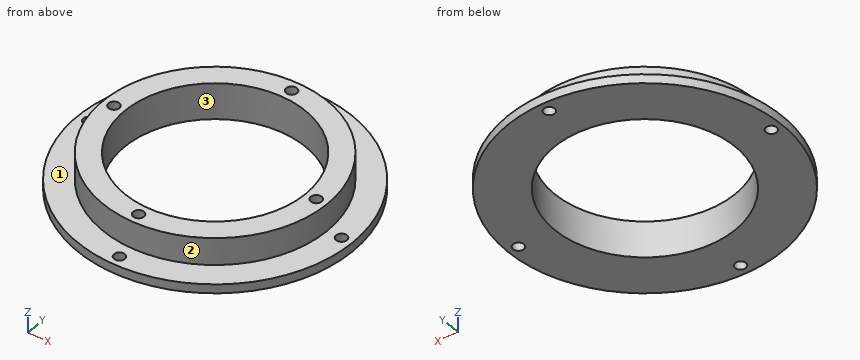
Autodesk Inventor part; units mm, degrees
ref_plane "YZ Plane" through (0, 0, 0) normal (1, 0, 0) x (0, 1, 0)
ref_plane "XZ Plane" through (0, 0, 0) normal (0, 1, 0) x (-1, 0, 0)
ref_plane "XY Plane" through (0, 0, 0) normal (0, 0, 1) x (1, 0, 0)
sketch "스케치1" plane through (0, 0, 0) normal (0, 0, 1) x (1, 0, 0)
  circle A0 centre (0, 0) radius 25
  circle A1 centre (-35, 0) radius 1.5
  circle A2 centre (0, 0) radius 31
  circle A3 centre (0, 0) radius 38
  circle A4 centre (0, -35) radius 1.5
  circle A5 centre (35, 0) radius 1.5
  circle A6 centre (0, 35) radius 1.5
  dimension "d0" = 50
  dimension "d2" = 3
  dimension "d4" = 6
  dimension "d27" = 1.5
  dimension "d28" = 35
  dimension "d31" = 360
extrude "돌출1" add sketch "스케치1" along normal blind 2.5 contours A3
extrude "돌출2" add sketch "스케치1" along normal blind 10 contours A2
sketch "스케치2" plane through (0, 0, 10) normal (0, 0, 1) x (1, 0, 0)
  circle A0 centre (0, 0) radius 25
  circle A1 centre (0, 0) radius 31
  line L0 (-1.611, 31) -> (1.611, 31)
  point P0 (0, 28)
  point P1 (0, 31)
  point P2 (-28, 0)
  point P3 (0, -28)
  point P4 (28, 0)
  dimension "d14" = 6
  dimension "d15" = 3
  dimension "d18" = 360
hole "구멍1" at (0, 28, 10) at (-28, 0, 10) at (0, -28, 10) at (28, 0, 10) direction (0, 0, -1) diameter 3 depth 8 tip angle 118
properties part number "ModuleConnector"
Source: CAD feature listing. Evaluate the final solid. Frame: model axes, mm. Face numbers are marked on the shaded views. Coordinates: 2 decimals unless noted, no trailing zeros. Loops run counter-clockwise (first coordinate to the right, second up) from the corner with the lowest first, then second, coordinate; pieces in that order, holes last. Notation, with made-up numbers: M 63,20.25 L 85,20.25 A17 cw 85,29.25 Z; hole C 64.25,61.5 d11. An arc over 180 degrees is marked long. Use CSV: the item, a comma, the result in double quotes.
(1) Cut plane A-A on x = 23.5. Return loops of the section in (y, z).
Answers follow:
outline,"M -29.86,0 L -8.53,0 L -8.53,10 L -20.22,10 L -20.22,2.5 L -29.86,2.5 Z; M 8.53,0 L 29.86,0 L 29.86,2.5 L 20.22,2.5 L 20.22,10 L 8.53,10 Z"
(2) Contact query for flat-ended pins moving along their axis: pin 1 (5 mm diameter, centred on y = 20, z = 4.5, fed in from +X); pin 2 (3 mm diameter, centred on y = 11.5, z = 5.5, fed in from -X); pin 3 (1.8 mm diameter, centred on x = 0, y = 28, fed in from +Z). Output: stop coordinate, or through.
Answers follow:
pin 1,"x = 33.19"
pin 2,"x = -29.34"
pin 3,"z = 1.64"
(3) Line query: line 1 (Y direction, x = 0, z = 7.25); line 2 (Y direction, x = 0, z = 1.4); line 3 (Z direction, x = 26, y = 25). Output: solid intervals per line, ascending. Write a range as [from, to].
Answers follow:
line 1,"[-31, -29.5], [-26.5, -25], [25, 26.5], [29.5, 31]"
line 2,"[-38, -36.5], [-33.5, -28.5], [-27.5, -25], [25, 27.5], [28.5, 33.5], [36.5, 38]"
line 3,"[0, 2.5]"
(4) Cut plane C-C on z = 4.5. Return loops of the section in (x, y), and give its area (3 significant figures).
Answers follow:
outline,"C 0,0 d62; hole C -28,0 d3; hole C 0,0 d50; hole C 0,-28 d3; hole C 0,28 d3; hole C 28,0 d3"
area,"1,030 mm²"
(5) Cut plane D-D on x = 11. Return loops of the section in (y, z), and give its area (3 significant figures).
Answers follow:
outline,"M -36.37,0 L -22.45,0 L -22.45,10 L -28.98,10 L -28.98,2.5 L -36.37,2.5 Z; M 22.45,0 L 36.37,0 L 36.37,2.5 L 28.98,2.5 L 28.98,10 L 22.45,10 Z"
area,"168 mm²"
(6) Draft query along X for the marked faces 1, 2 and 3. Return one class per face: pulls with the +X half, pulls with the -X half, needs draft (parallel to the pull), parting line crosses it, or undercut.
Answers follow:
face 1,"needs draft"
face 2,"parting line crosses it"
face 3,"undercut"
(7) Cut plane B-B on y = 35. Return loops of the section in (x, z), and give its area (3 significant figures).
Answers follow:
outline,"M -14.8,0 L -1.5,0 L -1.5,2.5 L -14.8,2.5 Z; M 1.5,0 L 14.8,0 L 14.8,2.5 L 1.5,2.5 Z"
area,"66.5 mm²"
